Source: three-view drawing plus pictorial views. Frame: mm from the lowest corner of the part. Coordinates: 2 decimals unless noted, no trailing zeros. Write each loop counter-clockwise with the first axis right and the second up, starting at its lowest first coordinate (ties: lowest second). Pieces come first, ordered by that corner, then holes. Notation, with made-up numbers: (1.5, 32.25) - (21.5, 32.25) arc R26 cw to (21.5, 57.25) - close; hole circle Ø8 at (47, -3). An arc over 180 degrees is marked (long way). One line per item, written item: value.
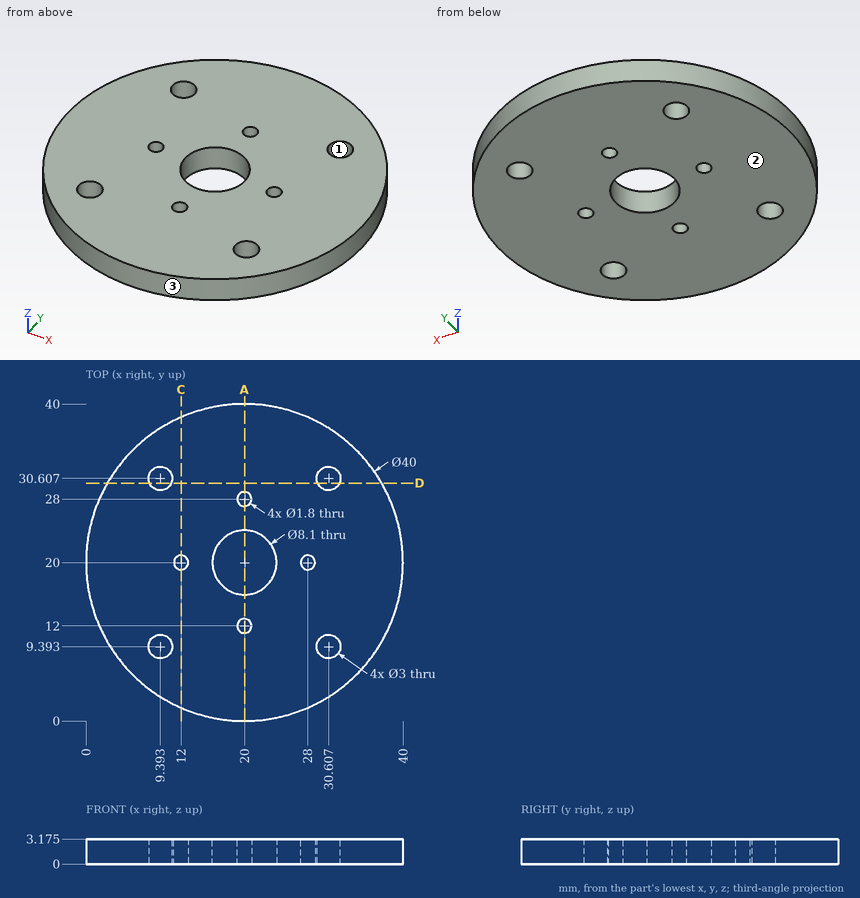
1) Section query A-A on x = 20. State how many separate pieces and enclosed holes the cut face has.
Values found:
separate pieces: 4
enclosed holes: 0
2) Material intervals for line 1 (Y direction, x = 20, z = 2.45); line 2 (X direction, y = 9, z = 2.3) (1 decimal); line 3 (X direction, y = 8.5, z = 0.25) (1 decimal), sorted ascending.
Values found:
line 1: 0 to 11.1, 12.9 to 15.95, 24.05 to 27.1, 28.9 to 40
line 2: 3.3 to 7.9, 10.8 to 29.2, 32.1 to 36.7
line 3: 3.6 to 8.2, 10.6 to 29.4, 31.8 to 36.4
3) Section query D-D on y = 30. Output: boundary loops of the cut face in (x, z) (1 decimal).
Values found:
outline: (2.7, 0) - (8, 0) - (8, 3.2) - (2.7, 3.2) - close; (10.8, 0) - (29.2, 0) - (29.2, 3.2) - (10.8, 3.2) - close; (32, 0) - (37.3, 0) - (37.3, 3.2) - (32, 3.2) - close
4) Draft query along X for the marked faces 1, 2 and 3. Return one class per face: released by +X, released by -X, zero draft, split by the parting line, or undercut.
Values found:
face 1: undercut
face 2: zero draft
face 3: split by the parting line
5) Contact query for a flat-ended pin moving along its axis: P1, Ø2.5, axis at x = 12, y = 20, coming from the +Z side (3 decimals). Output: stop coordinate, or through.
Values found:
P1: z = 3.175
6) Section query C-C on x = 12. Output: boundary loops of the cut face in (y, z) (1 decimal), then the cut area to 3 significant figures.
Values found:
outline: (1.7, 0) - (19.1, 0) - (19.1, 3.2) - (1.7, 3.2) - close; (20.9, 0) - (38.3, 0) - (38.3, 3.2) - (20.9, 3.2) - close
area: 111 mm2
